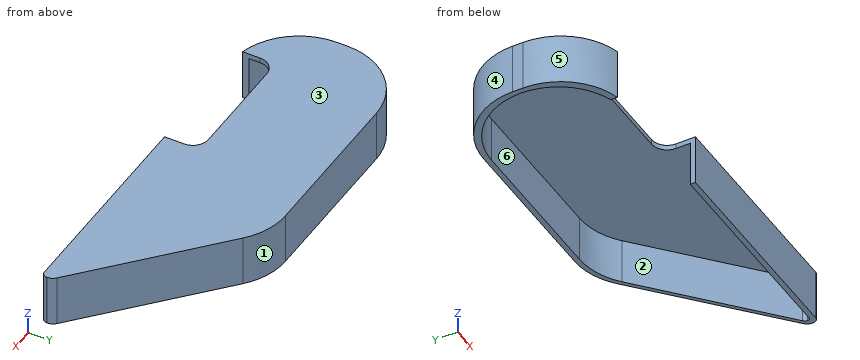
from build123d import *

# Parameters (mm, degrees)
SKETCH1_W               = 80
SKETCH1_H               = 30
BOSS_EXTRUDE1_DEPTH     = 10
CUT_EXTRUDE2_DEPTH      = 87.02325267
CUT_EXTRUDE2_DEPTH_BACK = 10
SKETCH9_OUTSIDE_W       = 99.204
SKETCH9_OUTSIDE_H       = 49.204
CUT_EXTRUDE3_DEPTH      = 10
CUT_EXTRUDE5_DEPTH      = 9
FILLET13_R              = 13
FILLET14_R              = 13
FILLET15_R              = 13
FILLET17_R              = 13
FILLET18_R              = 13
FILLET19_R              = 13
FILLET20_R              = 2
FILLET21_R              = 1
FILLET22_R              = 0.5
FILLET23_R              = 1
SKETCH15_W              = 26
SKETCH15_H              = 7
CUT_EXTRUDE6_DEPTH      = 15
FILLET24_R              = 3
FILLET25_R              = 3


with BuildPart() as part:
    # Sketch1 → Boss-Extrude1 (new body)
    with BuildSketch(Plane.XY):
        with Locations((40, 15)):
            Rectangle(SKETCH1_W, SKETCH1_H)
    extrude(amount=BOSS_EXTRUDE1_DEPTH)

    # Sketch2 → Cut-Extrude2 (cut, two sides: drawn at the far end of the back side and taken through both)
    with BuildSketch(Plane.XY.offset(10).offset(-CUT_EXTRUDE2_DEPTH_BACK)):
        Polygon((50, 30), (80, 3), (80, 30), align=None)
    extrude(amount=CUT_EXTRUDE2_DEPTH + CUT_EXTRUDE2_DEPTH_BACK, mode=Mode.SUBTRACT)

    # Sketch9 outside → Cut-Extrude3 (cut)
    with BuildSketch(Plane.XY.offset(10)):
        with Locations((40, 15)):
            Rectangle(SKETCH9_OUTSIDE_W, SKETCH9_OUTSIDE_H)
        Polygon((1.004393743, 1.037027121), (79.0058654, 0.993658775), (79.0058654, 3), (50, 29.001260854), (1.004393743, 28.998403262), align=None, mode=Mode.SUBTRACT)
    extrude(amount=-CUT_EXTRUDE3_DEPTH, mode=Mode.SUBTRACT)

    # Sketch14 → Cut-Extrude5 (cut)
    with BuildSketch(Plane(origin=(0, 0, 0), x_dir=(-1, 0, 0), z_dir=(0, 0, -1))):
        Polygon((-50, 28.003177056), (-2.012705642, 28.003177056), (-2.00811371, 2.035465522), (-78.002698254, 1.991852338), (-78.002698254, 3), align=None)
    extrude(amount=-CUT_EXTRUDE5_DEPTH, mode=Mode.SUBTRACT)

    # Fillet13
    fillet13_edges = [part.edges().sort_by_distance(p)[0] for p in [
        (2.012705642, 28.003177056, 4.5),
    ]]
    fillet(fillet13_edges, radius=FILLET13_R)

    # Fillet14
    # the kernel refuses this fillet: 13 mm, written as the material it adds along each edge
    with BuildSketch(Plane(origin=(2.00811371, 2.035465522, 0), x_dir=(0.0001768323716472033, 0.999999984365156, 0), z_dir=(0, 0, 1))) as fillet14_piece_1:
        with BuildLine():
            CenterArc((FILLET14_R * 0.999603012675, -FILLET14_R), FILLET14_R, 90, 89.977249786)
            Line((-FILLET14_R * 0.000396908494235, -FILLET14_R * 0.999602933876), (0, 0))
            Line((0, 0), (FILLET14_R * 0.999603012675, 0))
        make_face()
    extrude(amount=9)

    # Fillet15
    fillet15_edges = [part.edges().sort_by_distance(p)[0] for p in [
        (50, 28.003177056, 4.5),
    ]]
    fillet(fillet15_edges, radius=FILLET15_R)

    # Fillet17
    fillet17_edges = [part.edges().sort_by_distance(p)[0] for p in [
        (1.004393743, 28.998403262, 5),
    ]]
    fillet(fillet17_edges, radius=FILLET17_R)

    # Fillet18
    fillet18_edges = [part.edges().sort_by_distance(p)[0] for p in [
        (1.004393743, 1.037027121, 5),
    ]]
    fillet(fillet18_edges, radius=FILLET18_R)

    # Fillet19
    fillet19_edges = [part.edges().sort_by_distance(p)[0] for p in [
        (50, 29.001260854, 5),
    ]]
    fillet(fillet19_edges, radius=FILLET19_R)

    # Fillet20
    fillet20_edges = [part.edges().sort_by_distance(p)[0] for p in [
        (79.0058654, 3, 5),
    ]]
    fillet(fillet20_edges, radius=FILLET20_R)

    # Fillet21
    fillet21_edges = [part.edges().sort_by_distance(p)[0] for p in [
        (79.0058654, 0.993658775, 5),
    ]]
    fillet(fillet21_edges, radius=FILLET21_R)

    # Fillet22
    fillet22_edges = [part.edges().sort_by_distance(p)[0] for p in [
        (78.002698254, 1.991852338, 4.5),
    ]]
    fillet(fillet22_edges, radius=FILLET22_R)

    # Fillet23
    fillet23_edges = [part.edges().sort_by_distance(p)[0] for p in [
        (78.002698254, 3, 4.5),
    ]]
    fillet(fillet23_edges, radius=FILLET23_R)

    # Sketch15 → Cut-Extrude6 (cut)
    with BuildSketch(Plane.XY.offset(10)):
        with Locations((24.004393743, 4.300352014)):
            Rectangle(SKETCH15_W, SKETCH15_H)
    extrude(amount=-CUT_EXTRUDE6_DEPTH, mode=Mode.SUBTRACT)

    # Fillet24
    fillet24_edges = [part.edges().sort_by_distance(p)[0] for p in [
        (11.004393743, 7.800352014, 9.5),
    ]]
    fillet(fillet24_edges, radius=FILLET24_R)

    # Fillet25
    fillet25_edges = [part.edges().sort_by_distance(p)[0] for p in [
        (37.004393743, 7.800352014, 9.5),
    ]]
    fillet(fillet25_edges, radius=FILLET25_R)


solid = part.part
Check sheet for the modelled part. Datum: model origin and axes. Units: mm. Face numbers are marked on the shaded views. A direction names the side the tool comes from. Round coordinates to 2 decimals unless told otherwise and drop trailing zeros. Loops run counter-clockwise (first coordinate to the right, second up) from the corner with the lowest first, then second, coordinate; pieces in that order, holes last. Notation, with made-up numbers: (0, 42.5) -> (26, 42.5) arc R24 ccw to (26, 76.5) -> close; hole circle Ø2 at (18.5, 53). An arc over 180 degrees is marked (long way). Put each result on its own line as item: value. Start each with the question number.
1. Section check C-C (x = 41). Enter the section's corners in (y, z).
2. Section check B-B (z = 6.5). Enter the section's corners in (x, y), plus the area to 3 significant figures.
3. Gauge pin test, flat ends, axial feed: pin 1 (6 mm diameter, centred on y = 24, z = 1, fed in from -X); pin 2 (6 mm diameter, centred on x = 13, z = 1, fed in from -Y); pin 3 (4.5 mm diameter, centred on x = 34, z = 6.5, fed in from -Y). Record the tip position at first contact, or that the pin passes through.
4. Draft check along X on the marked faces 1, 2, 3 and 4. Enter one of: +X half, -X half, draft (parallel to the pull), parting line (faces both ways), or undercut.
5. Section check D-D (y = 21.75). Enter the section's corners in (x, z).
6. Scan lines: probe 1 along Y at (x, z) = (44, 2.25); probe 2 along Y at (x, z) = (47, 3); probe 3 along X at (y, z) = (6.5, 2.5). Record each from-to range of solid material in increasing order.
7. Access from +Z, -Z, +X, -X, +Y, -Y to the whole of each face (thin tool, end or side, straight path). Record for the marked faces 5 and 6.
8. Section check A-A (y = 6). Enter the section's corners in (x, z).
Findings:
1. outline: (1.01, 0) -> (2.01, 0) -> (2.01, 9) -> (28, 9) -> (28, 0) -> (29, 0) -> (29, 10) -> (1.01, 10) -> close
2. outline: (1, 14.03) arc R13 ccw to (11, 1.38) -> (11, 2.66) arc R13 cw to (2.01, 15.02) arc R13 cw to (15.01, 28) -> (45.04, 28) arc R13 cw to (53.7, 24.7) -> (77.67, 3.3) arc R1 cw to (78, 2.55) -> (78, 2.49) arc R0.5 cw to (77.5, 1.99) -> (37, 2.02) -> (37, 1.02) -> (78.01, 0.99) arc R1 ccw to (79.01, 1.99) -> (79.01, 2.11) arc R2 ccw to (78.34, 3.6) -> (53.7, 25.68) arc R13 ccw to (45.03, 29) -> (14, 29) arc R13 ccw to (1, 16) -> close
2. area: 154 mm^2
3. pin 1: stops at x = 2
3. pin 2: stops at y = 1.38
3. pin 3: stops at y = 28
4. face 1: +X half
4. face 2: undercut
4. face 3: draft
4. face 4: -X half
5. outline: (2.35, 0) -> (3.9, 0) -> (3.9, 9) -> (57, 9) -> (57, 0) -> (58.09, 0) -> (58.09, 10) -> (2.35, 10) -> close
6. probe 1: y = 1.01 to 2.01, 28 to 29
6. probe 2: y = 1.01 to 2.01, 27.85 to 28.85
6. probe 3: x = 3.41 to 5.2, 74.08 to 75.1
7. face 5: +Z, -Z, -X, -Y
7. face 6: -Z
8. outline: (3.78, 0) -> (5.66, 0) -> (5.66, 9) -> (11.25, 9) -> (11.25, 10) -> (3.78, 10) -> close; (36.75, 9) -> (74.64, 9) -> (74.64, 0) -> (75.66, 0) -> (75.66, 10) -> (36.75, 10) -> close
